Autodesk Inventor part; units mm, degrees
ref_plane "Work Plane1" through (5, 4.9851, -4.9851) normal (0, 0.7071068, -0.7071068) x (-1, 0, 0)
ref_plane "YZ Plane" through (0, 0, 0) normal (1, 0, 0) x (0, 1, 0)
ref_plane "XZ Plane" through (0, 0, 0) normal (0, 1, 0) x (-1, 0, 0)
sketch "Sketch1" plane through (0, 0, 0) normal (1, 0, 0) x (0, 1, 0)
  circle A0 centre (0, 0) radius 3.05
  circle A1 centre (0, 0) radius 7.05
  dimension "d0" = 6.1
  dimension "d1" = 4
extrude "Extrusion1" add sketch "Sketch1" along normal blind 5
sketch "Sketch2" plane through (5, 0, 0) normal (1, 0, 0) x (0, 0, -1)
  line L0 (0, 0) -> (4.9851, 4.9851)
  circle A0 centre (0, 0) radius 7.05
  line L1 (0, 0) -> (7.05, 0) construction
  dimension "d4" = 45
ref_plane "Work Plane1" through (5, 4.9851, -4.9851) normal (0, 0.7071068, -0.7071068) x (-1, 0, 0)
sketch "Sketch3" plane through (5, 4.9851, -4.9851) normal (0, 0.7071068, -0.7071068) x (-1, 0, 0)
  line L0 (5, 0) -> (0, 0)
  line L1 (0, 7.05) -> (0, -7.05)
  line L2 (5, 0) -> (10, 0) construction
  circle A0 centre (2.5, 0) radius 1.5
  dimension "d5" = 5
  dimension "d6" = 180
  dimension "d7" = 3
extrude "Extrusion2" cut sketch "Sketch3" against normal blind 5
thread "Thread1"
fillet "Fillet1" radius 2 2 edges at (5, -7.05, 0) (0, -7.05, 0)
properties part number "6mm rod topper"
The listing builds one solid part. Answer for the finished solid, in the listing's coordinates (mm). Give positions to 0.01 mm unless a question says otherwise; leave off trailing zeros. Order: outer loops, then holes, each group sorted by start corner. A loop starts at its lowest first (then second) coordinate and runs counter-clockwise, first axis right, second up. Notation, with made-up numbers: (-8.5, 8.5) - (6.5, 8.5) arc R18 ccw to (6.5, 17.5) - close; hole circle Ø9 at (81.5, 14.25). An arc over 180 degrees is marked (long way). One line per item, written item: value. Start each with the question number.
1) Given pin 1 Ø3 at (x, z) = (4, 4) entering from +Y; pin 2 Ø6 at (y, z) = (-3, 5.5) entering from +X; pin 3 Ø2 at (x, z) = (3.5, 4.5) entering from +Y, each flat-ended and moving along its own axis, determine where each tip first touches the part or whether it passes through.
2) The mould has two halves that part along Z. Classify faces 1 (the face through (5, -0.1, -3.3)), 2 (the face through (4, 3, -3)), 3 (the face through (2.493, -5.186, 4.776)): released by +Z, released by -Z, zero draft, split by the parting line, or undercut.
3) A cutting plane is placed at D-D on x = 3.35. Give the vertices of the cut face in (y, z).
4) A cutting plane is placed at A-A on y = 0. Give the vertices of the cut face in (x, z), then the cut area to 3 significant figures.
5) A cutting plane is placed at C-C on x = 0.6. Give the vertices of the cut face in (y, z).
6) Find the intervals of material crossed by L1, parallel to Z at x = 2.9, y = 0; L2, parallel to Z at x = 3.65, y = 0; L3, parallel to Y at x = 4.2, z = 1.25, in increasing order.
Answer sheet:
1. pin 1: stops at y = 6.5
1. pin 2: stops at x = 5
1. pin 3: stops at y = 6.08
2. face 1: zero draft
2. face 2: undercut
2. face 3: split by the parting line
3. outline: (1.1, -2.85) arc R3.05 cw (long way) to (2.85, -1.1) - (5.76, -4.01) arc R7.02 ccw (long way) to (4.01, -5.76) - close
4. outline: (0, -5.05) arc R2 ccw to (2, -7.05) - (3, -7.05) arc R2 ccw to (5, -5.05) - (5, -3.05) - (0, -3.05) - close; (0, 3.05) - (5, 3.05) - (5, 5.05) arc R2 ccw to (3, 7.05) - (2, 7.05) arc R2 ccw to (0, 5.05) - close
4. area: 36.6 mm2
5. outline: circle Ø12.96 at (0, 0); hole circle Ø6.1 at (0, 0)
6. L1: z = -7.05 to -3.05, 3.05 to 7.05
6. L2: z = -6.94 to -3.05, 3.05 to 6.94
6. L3: y = -6.53 to -2.78, 2.78 to 6.53
